from build123d import *

# Parameters (mm, degrees)
SM_BASE_FLANGE_1_DEPTH = 374
SKETCH_6_R             = 2.5
SKETCH_6_W             = 6.5
SKETCH_6_H             = 15
CUT_EXTRUDE_1_DEPTH    = 376.851366899
SKETCH_7_W             = 50
SKETCH_7_H             = 70
CUT_EXTRUDE_2_DEPTH    = 5


# Sheet-metal steps are written as plain solids
with BuildPart() as part:
    # Sketch 1 → Базовая кромка1 (new, symmetric)
    with BuildSketch(Plane.XY):
        with BuildLine():
            Line((-22.5, -27), (-22.5, -1.5))
            ThreePointArc((-22.5, -1.5), (-22.060660172, -0.439339828), (-21, 0))
            Line((-21, 0), (21, 0))
            ThreePointArc((21, 0), (22.060660172, -0.439339828), (22.5, -1.5))
            Line((22.5, -1.5), (22.5, -27))
            Line((22.5, -27), (24, -27))
            Line((24, -27), (24, -1.5))
            ThreePointArc((24, -1.5), (23.121320344, 0.621320344), (21, 1.5))
            Line((21, 1.5), (-21, 1.5))
            ThreePointArc((-21, 1.5), (-23.121320344, 0.621320344), (-24, -1.5))
            Line((-24, -1.5), (-24, -27))
            Line((-24, -27), (-22.5, -27))
        make_face()
    extrude(amount=SM_BASE_FLANGE_1_DEPTH, both=True)

    # Эскиз6 → Вырез-Вытянуть1 (cut, through all)
    with BuildSketch(Plane(origin=(0, 1.5, 0), x_dir=(1, 0, 0), z_dir=(0, 1, 0))):
        with Locations(Location((0, -360, 0), (0, 0, 180))):
            Circle(SKETCH_6_R)
        with Locations((0, 360)):
            Circle(SKETCH_6_R)
        with Locations((-21.75, -366.5)):
            Rectangle(SKETCH_6_W, SKETCH_6_H)
        with Locations((21.75, -366.5)):
            Rectangle(SKETCH_6_W, SKETCH_6_H)
        with Locations((21.75, 366.5)):
            Rectangle(SKETCH_6_W, SKETCH_6_H)
        with Locations((-21.75, 366.5)):
            Rectangle(SKETCH_6_W, SKETCH_6_H)
    extrude(amount=-CUT_EXTRUDE_1_DEPTH, mode=Mode.SUBTRACT)

    # Эскиз7 → Вырез-Вытянуть2 (cut)
    with BuildSketch(Plane(origin=(0, 1.5, 0), x_dir=(1, 0, 0), z_dir=(0, 1, 0))):
        with Locations((0, -293.5)):
            Rectangle(SKETCH_7_W, SKETCH_7_H)
        with Locations((0, 293.5)):
            Rectangle(SKETCH_7_W, SKETCH_7_H)
    extrude(amount=-CUT_EXTRUDE_2_DEPTH, mode=Mode.SUBTRACT)


solid = part.part
Work out the finished part from the listing and answer in its coordinate system (mm). A direction names the side the tool comes from. Round coordinates to 2 decimals unless told otherwise and drop trailing zeros. Loops run counter-clockwise (first coordinate to the right, second up) from the corner with the lowest first, then second, coordinate; pieces in that order, holes last. Notation, with made-up numbers: (-40, 70) - (8, 70) arc R26 cw to (8, 93) - close; hole circle Ø6 at (-15.75, 38). An arc over 180 degrees is marked (long way). Use one line per item in the form item = value. Start each with the question number.
(1) Consider line 1 (Z direction, x = 0, y = 1.15); line 2 (X direction, y = -22, z = -13); line 3 (X direction, y = 1.25, z = 360). Determine where each line is inside the solid, lowest interval first.
(2) Which of the six approach directions +Z, -Z, +X, -X, +Y, -Y give full straight-line access (tool end or side, diameter ignored) to faces 1 (the face through (0, 0, 4)), 2 (the face through (24, -14, 5))?
(3) Flat-ended cylindrical pins translate along their axes: P1, Ø12, axis at x = -14.5, y = -8.5, coming from the +Z side; P2, Ø12.5, axis at x = 10, z = 361.5, coming from the -Y side; P3, Ø1.6, axis at x = 23, z = 277, coming from the +Y side; P4, Ø0.8, axis at y = 1, z = -368.5, coming from the +X side. Find the tip coordinate at first contact, or state that the pin passes through.
(4) Find section B-B on z = -225. Determine the outline of the cut face in (x, y).
(5) Determine the mould class of faces 3 (the face through (0, 1.5, 352)), 4 (the face through (-22.5, -14, 5)), 5 (the face through (-24, -14, 5)) for opening direction X: +X half, -X half, draft (parallel to the pull), parting line (faces both ways), or undercut.
(6) Find section A-A on y = -14.75. Determine the outline of the cut face in (x, z), and give its area (3 significant figures).
Answer list:
q1.line_1 = -374 to -362.5, -357.5 to -328.5, -258.5 to 258.5, 328.5 to 357.5, 362.5 to 374
q1.line_2 = -24 to -22.5, 22.5 to 24
q1.line_3 = -18.5 to -2.5, 2.5 to 18.5
q2.face_1 = +Z, -Z, -Y
q2.face_2 = +Z, -Z, +X, +Y, -Y
q3.P1 = through
q3.P2 = 0
q3.P3 = -3.5
q3.P4 = 18.5
q4.outline = (-24, -27) - (-22.5, -27) - (-22.5, -1.5) arc R1.5 cw to (-21, 0) - (21, 0) arc R1.5 cw to (22.5, -1.5) - (22.5, -27) - (24, -27) - (24, -1.5) arc R3 ccw to (21, 1.5) - (-21, 1.5) arc R3 ccw to (-24, -1.5) - close
q5.face_3 = draft
q5.face_4 = undercut
q5.face_5 = -X half
q6.outline = (-24, -359) - (-22.5, -359) - (-22.5, 359) - (-24, 359) - close; (22.5, -359) - (24, -359) - (24, 359) - (22.5, 359) - close
q6.area = 2,150 mm^2
